```python
from build123d import *

# Parameters (mm, degrees)
EXTRUDE_THIN1_DEPTH             = 609.6
F_1_4_0_25_DIAMETER_HOLE1_D     = 6.35
F_1_4_0_25_DIAMETER_HOLE1_DEPTH = 25.4
F_1_4_0_25_DIAMETER_HOLE1_TIP   = 1.907732465


with BuildPart() as part:
    # Sketch1 → Extrude-Thin1 (new, symmetric)
    with BuildSketch(Plane.XY):
        with BuildLine():
            Line((-10, -7.5), (-10, 7.5))
            ThreePointArc((-10, 7.5), (-9.267766953, 9.267766953), (-7.5, 10))
            Line((-7.5, 10), (7.5, 10))
            ThreePointArc((7.5, 10), (9.267766953, 9.267766953), (10, 7.5))
            Line((10, 7.5), (10, -7.5))
            ThreePointArc((10, -7.5), (9.267766953, -9.267766953), (7.5, -10))
            Line((7.5, -10), (-7.5, -10))
            ThreePointArc((-7.5, -10), (-9.267766953, -9.267766953), (-10, -7.5))
        make_face()
        with BuildLine():
            Line((-8, -7.5), (-8, 7.5))
            ThreePointArc((-8, 7.5), (-7.853553391, 7.853553391), (-7.5, 8))
            Line((-7.5, 8), (7.5, 8))
            ThreePointArc((7.5, 8), (7.853553391, 7.853553391), (8, 7.5))
            Line((8, 7.5), (8, -7.5))
            ThreePointArc((8, -7.5), (7.853553391, -7.853553391), (7.5, -8))
            Line((7.5, -8), (-7.5, -8))
            ThreePointArc((-7.5, -8), (-7.853553391, -7.853553391), (-8, -7.5))
        make_face(mode=Mode.SUBTRACT)
    extrude(amount=EXTRUDE_THIN1_DEPTH, both=True)

    # 1/4 (0.25) Diameter Hole1
    with Locations(Plane(origin=(0, 10, 0), x_dir=(1, 0, 0), z_dir=(0, 1, 0))):
        with Locations((-0.2, 596.9), (-0.2, -596.9)):
            Hole(F_1_4_0_25_DIAMETER_HOLE1_D / 2, depth=F_1_4_0_25_DIAMETER_HOLE1_DEPTH)
            with Locations((0, 0, -(F_1_4_0_25_DIAMETER_HOLE1_DEPTH + F_1_4_0_25_DIAMETER_HOLE1_TIP / 2))):  # 118° drill point
                Cone(0, F_1_4_0_25_DIAMETER_HOLE1_D / 2, F_1_4_0_25_DIAMETER_HOLE1_TIP, mode=Mode.SUBTRACT)


solid = part.part
```
CAD build for the part. Positions are in the model's coordinates, mm. Coordinates: 2 decimals unless noted, no trailing zeros. Write each loop counter-clockwise with the first axis right and the second up, starting at its lowest first coordinate (ties: lowest second). Pieces come first, ordered by that corner, then holes. Notation, with made-up numbers: (-24, 79.25) -> (25, 79.25) arc R25 ccw to (25, 118.25) -> close; hole circle Ø7 at (-33.5, 76). An arc over 180 degrees is marked (long way). Use CSV: the item, a comma, the result in double quotes. Start each with the question number.
Item 1: Band-saw the part on C-C, the plane z = -374. Write the cut outline in (x, y), plus the area to 3 significant figures.
Item 2: Wall check: probe 1 along Z at (x, y) = (-0.2, -8.4) (3 decimals); probe 2 along Y at (x, z) = (-4.75, -485). Give the ranges that are in metal, low to high.
Item 3: Band-saw the part on B-B, the plane x = -0.2. Write the cut outline in (y, z) (3 decimals), plus the area to 3 significant figures.
Item 4: Band-saw the part on A-A, the plane y = -3.5. Write the cut outline in (x, z).
Response values:
1,outline,"(-10, -7.5) arc R2.5 ccw to (-7.5, -10) -> (7.5, -10) arc R2.5 ccw to (10, -7.5) -> (10, 7.5) arc R2.5 ccw to (7.5, 10) -> (-7.5, 10) arc R2.5 ccw to (-10, 7.5) -> close; hole (-8, -7.5) arc R0.5 ccw to (-7.5, -8) -> (7.5, -8) arc R0.5 ccw to (8, -7.5) -> (8, 7.5) arc R0.5 ccw to (7.5, 8) -> (-7.5, 8) arc R0.5 ccw to (-8, 7.5) -> close"
1,area,"139 mm2"
2,probe 1,"z = -609.6 to -600.075, -593.725 to 593.725, 600.075 to 609.6"
2,probe 2,"y = -10 to -8, 8 to 10"
3,outline,"(-10, -609.6) -> (-8, -609.6) -> (-8, -600.075) -> (-10, -600.075) -> close; (-10, -593.725) -> (-8, -593.725) -> (-8, 593.725) -> (-10, 593.725) -> close; (-10, 600.075) -> (-8, 600.075) -> (-8, 609.6) -> (-10, 609.6) -> close; (8, -609.6) -> (10, -609.6) -> (10, -600.075) -> (8, -600.075) -> close; (8, -593.725) -> (10, -593.725) -> (10, 593.725) -> (8, 593.725) -> close; (8, 600.075) -> (10, 600.075) -> (10, 609.6) -> (8, 609.6) -> close"
3,area,"4,830 mm2"
4,outline,"(-10, -609.6) -> (-8, -609.6) -> (-8, 609.6) -> (-10, 609.6) -> close; (8, -609.6) -> (10, -609.6) -> (10, 609.6) -> (8, 609.6) -> close"
